Could you check a few things on this model? Use its own coordinates, in mm. A direction names the side the tool comes from. Coordinates: 2 decimals unless noted, no trailing zeros. Loops run counter-clockwise (first coordinate to the right, second up) from the corner with the lowest first, then second, coordinate; pieces in that order, holes last. Notation, with made-up numbers: (-37, -36.75) - (-13, -36.75) arc R20 ccw to (-13, -9.75) - close; hole circle Ø6 at (-17, 49.25). An arc over 180 degrees is marked (long way). One line per question, with ' | ' between items. Start each with the question number.
1. Which directions (+Z, -Z, +X, -X, +Y, -Y) give clear straight access to the entire face, cutting with the end or side of a thin tool? Please do faces 1 (the flat face through (3, -3, 0)), 2 (the flat face through (-3.3, -5.6, 2.5)).
2. I want a section at B-B, the plane z = -7. Write out the boundary of the cut face in (x, y), then the cut area to 3 significant figures.
3. I want a section at A-A, the plane y = 0. Write out the boundary of the cut face in (x, z).
4. I'm going to push flat-ended pins straight in: P1, Ø4, axis at y = -3, z = -14, coming from the +X side; P2, Ø6, axis at y = -5, z = -10, coming from the -X side; P3, Ø1.5, axis at y = -3, z = -17.5, coming from the +X side. Where does each tip first touch, or does it pass through?
5. Please list where these lines run through material, in increasing order: L1, parallel to Z at x = -2, y = -5.5; L2, parallel to X at y = -3, z = -4.5; L3, parallel to Y at x = 2.25, z = -8. Write a range as [from, to].
from build123d import *

# Parameters (mm, degrees)
EXTRUDE_1_DEPTH     = 5.3
SKETCH_2_OUTSIDE_W  = 61.562
SKETCH_2_OUTSIDE_H  = 63.574
SKETCH_2_OUTSIDE_R  = 6.25
CUT_EXTRUDE_1_DEPTH = 12.254924848
CUT_EXTRUDE_1_DRAFT = -60
SKETCH_3_R          = 4
EXTRUDE_2_DEPTH     = 20
CHAMFER_1_SIZE      = 1


with BuildPart() as part:
    # Эскиз1 → Бобышка-Вытянуть1 (new body)
    with BuildSketch(Plane.XY):
        Polygon((0, 7.505553499), (-6.5, 3.75277675), (-6.5, -3.75277675), (0, -7.505553499), (6.5, -3.75277675), (6.5, 3.75277675), align=None)
    extrude(amount=EXTRUDE_1_DEPTH)


with BuildPart() as cut_extrude_1_tool:
    # Эскиз2 outside → Вырез-Вытянуть1 (with draft: the straight prism first)
    with BuildSketch(Plane.XY.offset(5.3)):
        Rectangle(SKETCH_2_OUTSIDE_W, SKETCH_2_OUTSIDE_H)
        Circle(SKETCH_2_OUTSIDE_R, mode=Mode.SUBTRACT)
    extrude(amount=-CUT_EXTRUDE_1_DEPTH)
    # Вырез-Вытянуть1: the draft: its side faces are tilted about the plane it starts from
    cut_extrude_1_sides = [cut_extrude_1_tool.faces().sort_by_distance(p)[0] for p in [
        (0, -31.787, -0.827462424),
        (30.781, 0, -0.827462424),
        (0, 31.787, -0.827462424),
        (-30.781, 0, -0.827462424),
        (-6.25, 0, -0.827462424),
    ]]
    draft(cut_extrude_1_sides, Plane.XY.offset(5.3), CUT_EXTRUDE_1_DRAFT)


with BuildPart() as part_1:
    add(part.part)

    # Вырез-Вытянуть1: cut by cut_extrude_1_tool
    add(cut_extrude_1_tool.part, mode=Mode.SUBTRACT)

    # Эскиз3 → Бобышка-Вытянуть2 (add)
    with BuildSketch(Plane(origin=(0, 0, 0), x_dir=(-1, 0, 0), z_dir=(0, 0, -1))):
        with Locations(Location((0, 0, 0), (0, 0, 180))):
            Circle(SKETCH_3_R)
    extrude(amount=EXTRUDE_2_DEPTH)

    # Фаска1
    chamfer_1_edges = [part_1.edges().sort_by_distance(p)[0] for p in [
        (-4, 0, -20),
    ]]
    chamfer(chamfer_1_edges, length=CHAMFER_1_SIZE)


solid = part_1.part
Results are:
1) face 1: -Z | face 2: +Z, -Z, -X, -Y
2) outline: circle Ø8 at (0, 0) | area: 50.3 mm2
3) outline: (-6.5, 0) - (-4, 0) - (-4, -19) - (-3, -20) - (3, -20) - (4, -19) - (4, 0) - (6.5, 0) - (6.5, 5.16) - (6.25, 5.3) - (-6.25, 5.3) - (-6.5, 5.16) - close
4) P1: stops at x = 3.87 | P2: stops at x = -3.46 | P3: stops at x = 3.31
5) L1: z = [0, 5.3] | L2: x = [-2.65, 2.65] | L3: y = [-3.31, 3.31]
